Geometry check sheet. Reference: the model listing, model coordinates, mm. A direction names the side the tool comes from. Give positions to 0.01 mm unless a question says otherwise; leave off trailing zeros. Loops run counter-clockwise (first coordinate to the right, second up) from the corner with the lowest first, then second, coordinate; pieces in that order, holes last. Notation, with made-up numbers: (19.25, 42) -> (74.25, 42) arc R16 ccw to (74.25, 52) -> close; hole circle Ø2 at (16.25, -37). An arc over 180 degrees is marked (long way). One line per question, with ' | ' between items.
from build123d import *

# Parameters (mm, degrees)
EXTRUDE_1_DEPTH     = 15
CUT_EXTRUDE_1_DEPTH = 12
SKETCH_4_W          = 15.2
SKETCH_4_H          = 2.9
CUT_EXTRUDE_2_DEPTH = 6.1
SKETCH_5_R          = 1.5
CUT_EXTRUDE_3_DEPTH = 50.879855653
SKETCH_8_R          = 2.5
CUT_EXTRUDE_4_DEPTH = 50.879855653
SKETCH_9_R          = 3.5
SKETCH_9_R_2        = 4
CUT_EXTRUDE_6_DEPTH = 1


with BuildPart() as part:
    # 草圖1 → 填料-伸長1 (new body)
    with BuildSketch(Plane.XY):
        with BuildLine():
            Line((-33, 30), (33, 30))
            ThreePointArc((33, 30), (36.535533906, 28.535533906), (38, 25))
            Line((38, 25), (38, -25))
            ThreePointArc((38, -25), (36.535533906, -28.535533906), (33, -30))
            Line((33, -30), (-33, -30))
            ThreePointArc((-33, -30), (-36.535533906, -28.535533906), (-38, -25))
            Line((-38, -25), (-38, 25))
            ThreePointArc((-38, 25), (-36.535533906, 28.535533906), (-33, 30))
        make_face()
    extrude(amount=EXTRUDE_1_DEPTH)

    # 草圖2 → 除料-伸長1 (cut)
    with BuildSketch(Plane.XY.offset(15)):
        with BuildLine():
            Line((-30.1, 27.1), (30.1, 27.1))
            ThreePointArc((30.1, 27.1), (33.635533906, 25.635533906), (35.1, 22.1))
            Line((35.1, 22.1), (35.1, -22.1))
            ThreePointArc((35.1, -22.1), (33.635533906, -25.635533906), (30.1, -27.1))
            Line((30.1, -27.1), (-30.1, -27.1))
            ThreePointArc((-30.1, -27.1), (-33.635533906, -25.635533906), (-35.1, -22.1))
            Line((-35.1, -22.1), (-35.1, 22.1))
            ThreePointArc((-35.1, 22.1), (-33.635533906, 25.635533906), (-30.1, 27.1))
        make_face()
    extrude(amount=-CUT_EXTRUDE_1_DEPTH, mode=Mode.SUBTRACT)

    # 草圖3 → 除料-旋轉1 (revolve, cut)
    with BuildSketch(Plane(origin=(0, 0, 0), x_dir=(1, 0, 0), z_dir=(0, 1, 0)), mode=Mode.PRIVATE) as cut_revolve_1_sk:
        Polygon((0, -3), (14.7, -3), (14.7, -1.9), (14.7, 0), (0, 0), (0, -1.9), align=None)
    revolve(cut_revolve_1_sk.sketch.rotate(Axis((0, 0, -11.605627028), (0, 0, 1)), 180), axis=Axis((0, 0, -11.605627028), (0, 0, 1)), mode=Mode.SUBTRACT)

    # 草圖4 → 除料-伸長2 (cut)
    with BuildSketch(Plane.XY.offset(15)):
        with Locations((0, 28.55)):
            Rectangle(SKETCH_4_W, SKETCH_4_H)
        with Locations((0, -28.55)):
            Rectangle(SKETCH_4_W, SKETCH_4_H)
    extrude(amount=-CUT_EXTRUDE_2_DEPTH, mode=Mode.SUBTRACT)

    # 草圖5 → 除料-伸長3 (cut, through all)
    with BuildSketch(Plane.XY.offset(3)):
        with BuildLine():
            ThreePointArc((-0.654309657, 17.693297569), (-0.88727257, 17.38969439), (-0.837322359, 17.010284867))
            Line((-0.837322359, 17.010284867), (1.162677641, 13.546183252))
            ThreePointArc((1.162677641, 13.546183252), (1.725099866, 14.279146165), (1.845690343, 13.36317055))
            Line((1.845690343, 13.36317055), (6.175817362, 15.86317055))
            ThreePointArc((6.175817362, 15.86317055), (6.408780275, 16.16677373), (6.358830064, 16.546183252))
            Line((6.358830064, 16.546183252), (4.358830064, 20.010284867))
            ThreePointArc((4.358830064, 20.010284867), (4.055226885, 20.24324778), (3.675817362, 20.193297569))
            Line((3.675817362, 20.193297569), (-0.654309657, 17.693297569))
        make_face()
        with BuildLine():
            Line((-14.312677641, -9.230284867), (-12.312677641, -5.766183252))
            ThreePointArc((-12.312677641, -5.766183252), (-13.228653256, -5.645592775), (-12.495690343, -5.08317055))
            Line((-12.495690343, -5.08317055), (-16.825817362, -2.58317055))
            ThreePointArc((-16.825817362, -2.58317055), (-17.205226885, -2.533220339), (-17.508830064, -2.766183252))
            Line((-17.508830064, -2.766183252), (-19.508830064, -6.230284867))
            ThreePointArc((-19.508830064, -6.230284867), (-19.558780275, -6.60969439), (-19.325817362, -6.913297569))
            Line((-19.325817362, -6.913297569), (-14.995690343, -9.413297569))
            ThreePointArc((-14.995690343, -9.413297569), (-14.616280821, -9.46324778), (-14.312677641, -9.230284867))
        make_face()
        with BuildLine():
            Line((15.15, -7.78), (11.15, -7.78))
            ThreePointArc((11.15, -7.78), (10.796446609, -7.926446609), (10.65, -8.28))
            Line((10.65, -8.28), (10.65, -13.28))
            ThreePointArc((10.65, -13.28), (10.796446609, -13.633553391), (11.15, -13.78))
            Line((11.15, -13.78), (15.15, -13.78))
            ThreePointArc((15.15, -13.78), (15.503553391, -13.633553391), (15.65, -13.28))
            Line((15.65, -13.28), (15.65, -8.28))
            ThreePointArc((15.65, -8.28), (15.503553391, -7.926446609), (15.15, -7.78))
        make_face()
        with Locations((-32.4, 19.4)):
            Circle(SKETCH_5_R)
        with Locations((32.4, 17.9)):
            Circle(SKETCH_5_R)
        with Locations(Location((-32.4, -19.4, 0), (0, 0, 180))):
            Circle(SKETCH_5_R)
        with Locations((32.4, -19.4)):
            Circle(SKETCH_5_R)
        with Locations((-32.4, 12.1)):
            Circle(SKETCH_5_R)
        with Locations(Location((32.4, 12.1, 0), (0, 0, 180))):
            Circle(SKETCH_5_R)
        with Locations((32.4, -12.1)):
            Circle(SKETCH_5_R)
        with Locations(Location((-32.4, -12.1, 0), (0, 0, 180))):
            Circle(SKETCH_5_R)
    extrude(amount=-CUT_EXTRUDE_3_DEPTH, mode=Mode.SUBTRACT)

    # 草圖8 → 除料-伸長4 (cut, through all)
    with BuildSketch(Plane.XY.offset(3)):
        with Locations((-21.9, -19.4)):
            Circle(SKETCH_8_R)
        with Locations((21.9, 16.9)):
            Circle(SKETCH_8_R)
        with Locations(Location((-21.9, 16.9, 0), (0, 0, 180))):
            Circle(SKETCH_8_R)
    extrude(amount=-CUT_EXTRUDE_4_DEPTH, mode=Mode.SUBTRACT)

    # 草圖9 → 除料-伸長6 (cut)
    with BuildSketch(Plane(origin=(0, 0, 0), x_dir=(-1, 0, 0), z_dir=(0, 0, -1))):
        with Locations((-21.9, 16.9)):
            Circle(SKETCH_9_R)
        with Locations((21.9, -19.4)):
            Circle(SKETCH_9_R)
        with Locations((21.9, 16.9)):
            Circle(SKETCH_9_R_2)
    extrude(amount=-CUT_EXTRUDE_6_DEPTH, mode=Mode.SUBTRACT)


solid = part.part
Item 1: Sectioned sample at A-A (z = 6.5). Record the cut outline in (x, y).
Result:
outline: (-38, -25) arc R5 ccw to (-33, -30) -> (33, -30) arc R5 ccw to (38, -25) -> (38, 25) arc R5 ccw to (33, 30) -> (-33, 30) arc R5 ccw to (-38, 25) -> close; hole (-35.1, -22.1) arc R5 ccw to (-30.1, -27.1) -> (30.1, -27.1) arc R5 ccw to (35.1, -22.1) -> (35.1, 22.1) arc R5 ccw to (30.1, 27.1) -> (-30.1, 27.1) arc R5 ccw to (-35.1, 22.1) -> close
Item 2: Sectioned sample at D-D (y = 1). Record the cut outline in (x, z), plus the area to 3 significant figures.
Result:
outline: (-38, 0) -> (-14.67, 0) -> (-14.67, 3) -> (-35.1, 3) -> (-35.1, 15) -> (-38, 15) -> close; (14.67, 0) -> (38, 0) -> (38, 15) -> (35.1, 15) -> (35.1, 3) -> (14.67, 3) -> close | area: 210 mm2
Item 3: Release check for a two-part mould opening along Y. For faces 5 (the face through (36, 29, 7)), 6 (the face through (-36, 0, 15)), 7 (the face through (-33.83, -12.55, 1.52)) record: pulls with the +Y half, pulls with the -Y half, needs draft (parallel to the pull), parting line crosses it, or undercut.
Result:
face 5: pulls with the +Y half | face 6: needs draft | face 7: undercut
Item 4: Sectioned sample at C-C (x = 21.9). Record the cut outline in (y, z).
Result:
outline: (-30, 0) -> (13.4, 0) -> (13.4, 1) -> (14.4, 1) -> (14.4, 3) -> (-27.1, 3) -> (-27.1, 15) -> (-30, 15) -> close; (19.4, 1) -> (20.4, 1) -> (20.4, 0) -> (30, 0) -> (30, 15) -> (27.1, 15) -> (27.1, 3) -> (19.4, 3) -> close
Item 5: Sectioned sample at B-B (y = -19.4). Record the cut outline in (x, z), plus the area to 3 significant figures.
Result:
outline: (-38, 0) -> (-33.9, 0) -> (-33.9, 3) -> (-35.1, 3) -> (-35.1, 15) -> (-38, 15) -> close; (-30.9, 0) -> (-25.4, 0) -> (-25.4, 1) -> (-24.4, 1) -> (-24.4, 3) -> (-30.9, 3) -> close; (-19.4, 1) -> (-18.4, 1) -> (-18.4, 0) -> (30.9, 0) -> (30.9, 3) -> (-19.4, 3) -> close; (33.9, 0) -> (38, 0) -> (38, 15) -> (35.1, 15) -> (35.1, 3) -> (33.9, 3) -> close | area: 263 mm2
Item 6: Set-up check for faces 1 (the face through (-33.67, 25.6, 9.08)), 2 (the face through (-24, 19, 1)), 3 (the face through (-2.179, -14.538, 1.479)), 4 (the face through (-7.6, 29, 12)): record each of +Z, -Z, +X, -X, +Y, -Y from which the full face is reachable in a straight line by a thin tool's end or side.
Result:
face 1: +Z | face 2: -Z | face 3: +Z, -Z | face 4: +Z, +Y, -Y
Item 7: Scan lines: probe 1 along Y at (x, z) = (32.4, 1.3); probe 2 along Y at (x, z) = (-32.4, 1.4); probe 3 along X at (y, z) = (6.5, 8.75). Record each from-to range of solid material in increasing order.
Result:
probe 1: -30 to -20.9, -17.9 to -13.6, -10.6 to 10.6, 13.6 to 16.4, 19.4 to 30 | probe 2: -30 to -20.9, -17.9 to -13.6, -10.6 to 10.6, 13.6 to 17.9, 20.9 to 30 | probe 3: -38 to -35.1, 35.1 to 38
Item 8: Depth check by flat-ended pin: pin 1 Ø4 at (x, y) = (-13.5, -5.5) entering from +Z; pin 2 Ø6.5 at (x, y) = (-22, 17.5) entering from -Z; pin 3 Ø1.4 at (y, z) = (-28.5, 12) entering from +X. Enter the tip coordinate at first touch or a pass-through.
Result:
pin 1: z = 3 | pin 2: z = 1 | pin 3: x = 37.14
